CAD build for the part. Positions are in the model's coordinates, mm. Face numbers are marked on the shaded views. A direction names the side the tool comes from. Give positions to 0.01 mm unless a question says otherwise; leave off trailing zeros. Write each loop counter-clockwise with the first axis right and the second up, starting at its lowest first coordinate (ties: lowest second). Pieces come first, ordered by that corner, then holes. Notation, with made-up numbers: (19.25, -18) - (56.25, -18) arc R11 cw to (56.25, -6) - close; hole circle Ø7 at (4.25, 11.25). An arc over 180 degrees is marked (long way). Answer as a JSON object with one key per item and string values.
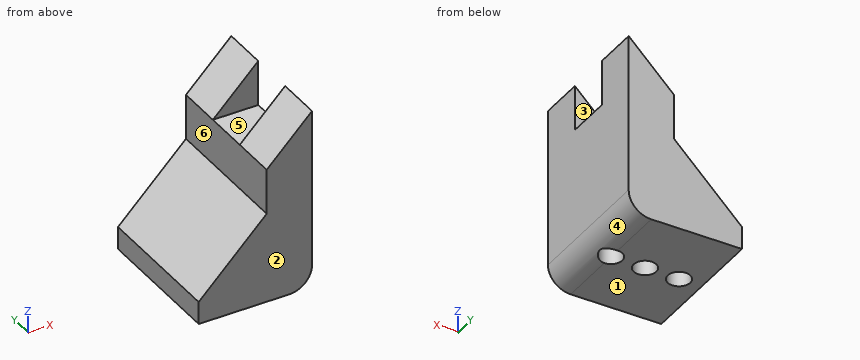
from build123d import *

# Parameters (mm, degrees)
F5_W        = 10
F5_H        = 10
F0_DEPTH    = 30
F1_DEPTH    = 10
F7_DEPTH    = 10
F3_D        = 5
F3_DEPTH    = 15
F3_TIP      = 1.5021515476
F8_D        = 5
F8_DEPTH    = 5
F8_TIP      = 1.5021515476
F4_T1_DEPTH = 55


# Not quite as in the source:
# - a fillet or chamfer that OpenCascade refuses, or shapes differently, is made with other operations: its cross-section is extruded or revolved along the edge and cut away or added


with BuildPart() as f0:
    # F5 (on Front) → F0 (new body)
    with BuildSketch(Plane.XZ):
        Polygon((10, 20), (10, 10), (20, 20), align=None)
        Polygon((20, 20), (10, 10), (20, 10), align=None)
        with Locations((15, 5)):
            Rectangle(F5_W, F5_H)
        Polygon((10, 10), (0, 0), (10, 0), align=None)
        Polygon((10, 0), (0, 0), (-5, -5), (-5, -10), (20, -10), (20, 0), align=None)
    extrude(amount=F0_DEPTH)

    # F5 (on Front) → F1 (join)
    with BuildSketch(Plane.XZ):
        Polygon((10, 20), (20, 20), (20, 30), align=None)
    extrude(amount=F1_DEPTH)

    # F6 (on face) → F7 (join)
    with BuildSketch(Plane.XZ.offset(30)):
        Polygon((10, 20), (20, 20), (20, 30), align=None)
    extrude(amount=-F7_DEPTH)

    # F3
    with Locations(Plane(origin=(0, 0, -10), x_dir=(1, 0, 0), z_dir=(0, 0, -1))):
        with Locations((15, 15)):
            Hole(F3_D / 2, depth=F3_DEPTH)
            with Locations((0, 0, -(F3_DEPTH + F3_TIP / 2))):  # 118° drill point
                Cone(0, F3_D / 2, F3_TIP, mode=Mode.SUBTRACT)

    # F8
    with Locations(Plane(origin=(0, 0, -10), x_dir=(1, 0, 0), z_dir=(0, 0, -1))):
        with Locations((7.5, 15), (0, 15)):
            Hole(F8_D / 2, depth=F8_DEPTH)
            with Locations((0, 0, -(F8_DEPTH + F8_TIP / 2))):  # 118° drill point
                Cone(0, F8_D / 2, F8_TIP, mode=Mode.SUBTRACT)

    # F4: fillet of radius 5 on 1 edges, made by hand

    # F4_s2 → F4_t1 (cut)
    with BuildSketch(Plane.XZ.offset(-12.5)):
        with BuildLine():
            ThreePointArc((20, -5), (18.5355339059, -8.5355339059), (15, -10))
            Line((15, -10), (20, -10))
            Line((20, -10), (20, -5))
        make_face()
    extrude(amount=F4_T1_DEPTH, mode=Mode.SUBTRACT)


solid = f0.part
(1) Pull direction Y, two halves, no side cores. Call the marked faces 1, 2 and 3: pulls with the +Y half, pulls with the -Y half, needs draft (parallel to the pull), parting line crosses it, or undercut.
Answer key:
{"face 1": "needs draft", "face 2": "pulls with the -Y half", "face 3": "undercut"}
(2) Saw through at D-D, the plane y = -18. Give the cut face in (x, z), and give its area (3 significant figures).
Answer key:
{"outline": "(-5, -10) - (15, -10) arc R5 ccw to (20, -5) - (20, 20) - (10, 20) - (10, 10) - (-5, -5) - close", "area": "482 mm²"}
(3) 3-axis set-ups, long thin cutter, end or side, ignore diameter. For the marked faces 4, 5 and 6: which of +Z, -Z, +X, -X, +Y, -Y reach the whole face in a straight line?
Answer key:
{"face 4": "-Z, +X, +Y, -Y", "face 5": "+Z, +X, -X", "face 6": "+Z, -X, +Y, -Y"}
(4) Flat gauge pins, fed straight in: P1, Ø4, axis at x = 7.5, y = -15, coming from the -Z side; P2, Ø8, axis at x = -2.5, y = -21, coming from the +Z side; P3, Ø8, axis at x = 16, z = 26.5, coming from the +Y side; P4, Ø6, axis at x = 1.5, z = 6.5, coming from the -Y side. Where does each tip first touch, or does it go through?
Answer key:
{"P1": "stops at z = -4.7", "P2": "stops at z = 1.5", "P3": "stops at y = 0", "P4": "passes through"}
(5) Saw through at B-B, the plane y = -5. Give the cut face in (x, z), and give its area (3 significant figures).
Answer key:
{"outline": "(-5, -10) - (15, -10) arc R5 ccw to (20, -5) - (20, 30) - (10, 20) - (10, 10) - (-5, -5) - close", "area": "532 mm²"}
(6) Saw through at A-A, the plane z = 3.5. Give the cut face in (x, y), and give its area (3 significant figures).
Answer key:
{"outline": "(3.5, -30) - (20, -30) - (20, 0) - (3.5, 0) - close; hole circle Ø5 at (15, -15)", "area": "475 mm²"}
(7) Probe L1, parallel to Y at x = 7.5, z = -7.45; L2, parallel to X at y = -15, z = -8.7; L3, parallel to X at y = -15, z = -7.3. List the from-to ranges inside material, lowest first. Write a range as [from, to].
Answer key:
{"L1": "y = [-30, -17.5], [-12.5, 0]", "L2": "x = [-5, -2.5], [2.5, 5], [10, 12.5], [17.5, 18.36]", "L3": "x = [-5, -2.5], [2.5, 5], [10, 12.5], [17.5, 19.44]"}
(8) Saw through at C-C, the plane z = 27. Give the cut face in (x, y), and give its area (3 significant figures).
Answer key:
{"outline": "(17, -30) - (20, -30) - (20, -20) - (17, -20) - close; (17, -10) - (20, -10) - (20, 0) - (17, 0) - close", "area": "60.0 mm²"}
